Read the model definition and answer for the solid it produces. Units are mm, in the model's axes. Coordinates: 2 decimals unless noted, no trailing zeros. Write each loop counter-clockwise with the first axis right and the second up, starting at its lowest first coordinate (ties: lowest second). Pieces come first, ordered by that corner, then holes.
(1) Straight lines are drawn through the part: line 1 along Z through (x, y) = (2, 1.65); line 2 along Z through (x, y) = (52, 2.2); line 3 along X through (y, z) = (1.9, -65) (3 decimals). For each, find the intervals that lie inside material, in ascending order.
(2) The part is cut by section A-A, the plane x = 30. Determine the outline of the cut face in (y, z), and give its area (3 significant figures).
(3) The part is cut by section B-B, the plane y = 2.5. State how many separate pieces and enclosed holes the cut face has, and give its area (3 significant figures).
(4) The part is cut by section D-D, the plane x = 51. Determine the outline of the cut face in (y, z).
(5) The part is cut by section C-C, the plane z = 1. Determine the outline of the cut face in (x, y), and give its area (3 significant figures).
(6) Given pin 1 (9.5 mm diameter, centred on x = 60, z = -60, fed in from -Y); pin 2 (1.5 mm diameter, centred on y = 1, z = -28.5, fed in from -X), each flat-ended and moving along its own axis, determine where each tip first touches the part or whether it passes through.
```python
from build123d import *

# Parameters (mm, degrees)
SKETCH_1_R          = 8
SKETCH_1_W          = 60
SKETCH_1_H          = 60
SKETCH_1_R_2        = 20
SKETCH_1_R_3        = 1.75
EXTRUDE_1_DEPTH     = 3
FILLET_1_R          = 10
CUT_EXTRUDE_START   = -3
SKETCH_2_R          = 6
CUT_EXTRUDE_1_DEPTH = 2
SKETCH_2_3_R        = 3.5
CUT_EXTRUDE_3_DEPTH = 97.213304693
CUT_EXTRUDE_6_DEPTH = 1.5


with BuildPart() as part:
    # Эскиз1 → Бобышка-Вытянуть1 (new body)
    # profile 1 of 5: a face of its own
    with BuildSketch(Plane(origin=(0, 0, 0), x_dir=(1, 0, 0), z_dir=(0, 1, 0))):
        with Locations((60, 60)):
            Circle(SKETCH_1_R)
    # profile 2 of 5: a face of its own
    with BuildSketch(Plane(origin=(0, 0, 0), x_dir=(1, 0, 0), z_dir=(0, 1, 0))):
        with Locations((0, 60)):
            Circle(SKETCH_1_R)
    # profile 3 of 5: a face of its own
    with BuildSketch(Plane(origin=(0, 0, 0), x_dir=(1, 0, 0), z_dir=(0, 1, 0))):
        with Locations((60, 0)):
            Circle(SKETCH_1_R)
    # profile 4 of 5: a face of its own
    with BuildSketch(Plane(origin=(0, 0, 0), x_dir=(1, 0, 0), z_dir=(0, 1, 0))):
        Circle(SKETCH_1_R)
    # profile 5 of 5: a face of its own
    with BuildSketch(Plane(origin=(0, 0, 0), x_dir=(1, 0, 0), z_dir=(0, 1, 0))):
        with Locations((30, 30)):
            Rectangle(SKETCH_1_W, SKETCH_1_H)
        with Locations(Location((30, 30, 0), (0, 0, 270))):
            Circle(SKETCH_1_R_2, mode=Mode.SUBTRACT)
        with Locations(Location((9, 51, 0), (0, 0, 270))):
            Circle(SKETCH_1_R_3, mode=Mode.SUBTRACT)
        with Locations(Location((51, 51, 0), (0, 0, 270))):
            Circle(SKETCH_1_R_3, mode=Mode.SUBTRACT)
        with Locations(Location((51, 9, 0), (0, 0, 270))):
            Circle(SKETCH_1_R_3, mode=Mode.SUBTRACT)
        with Locations(Location((9, 9, 0), (0, 0, 270))):
            Circle(SKETCH_1_R_3, mode=Mode.SUBTRACT)
    extrude(amount=EXTRUDE_1_DEPTH)

    # Скругление1
    fillet_1_edges = [part.edges().sort_by_distance(p)[0] for p in [
        (0, 1.5, -8),
        (0, 1.5, -52),
        (8, 1.5, -60),
        (52, 1.5, -60),
        (60, 1.5, -52),
        (60, 1.5, -8),
        (52, 1.5, 0),
        (8, 1.5, 0),
    ]]
    fillet(fillet_1_edges, radius=FILLET_1_R)

    # Эскиз2 → Вырез-Вытянуть1 (cut)
    with BuildSketch(Plane(origin=(0, 3, 0), x_dir=(1, 0, 0), z_dir=(0, 1, 0)).offset(CUT_EXTRUDE_START)):
        with Locations(Location((0, 60, 0), (0, 0, 270))):
            Circle(SKETCH_2_R)
        with Locations(Location((60, 60, 0), (0, 0, 270))):
            Circle(SKETCH_2_R)
        with Locations(Location((60, 0, 0), (0, 0, 270))):
            Circle(SKETCH_2_R)
        with Locations(Location((0, 0, 0), (0, 0, 270))):
            Circle(SKETCH_2_R)
    extrude(amount=CUT_EXTRUDE_1_DEPTH, mode=Mode.SUBTRACT)

    # Эскиз2<3> → Вырез-Вытянуть3 (cut, through all)
    with BuildSketch(Plane(origin=(0, 3, 0), x_dir=(1, 0, 0), z_dir=(0, 1, 0))):
        with Locations(Location((0, 0, 0), (0, 0, 270))):
            Circle(SKETCH_2_3_R)
        with Locations(Location((0, 60, 0), (0, 0, 270))):
            Circle(SKETCH_2_3_R)
        with Locations(Location((60, 60, 0), (0, 0, 270))):
            Circle(SKETCH_2_3_R)
        with Locations(Location((60, 0, 0), (0, 0, 270))):
            Circle(SKETCH_2_3_R)
    extrude(amount=-CUT_EXTRUDE_3_DEPTH, mode=Mode.SUBTRACT)

    # Эскиз5 → Вырез-Вытянуть6 (cut)
    with BuildSketch(Plane(origin=(0, 3, 0), x_dir=(1, 0, 0), z_dir=(0, 1, 0)).offset(CUT_EXTRUDE_START)):
        with BuildLine():
            Line((24.5, 57.5), (35.5, 57.5))
            ThreePointArc((35.5, 57.5), (36.914213562, 56.914213562), (37.5, 55.5))
            Line((37.5, 55.5), (37.5, 54.5))
            ThreePointArc((37.5, 54.5), (36.914213562, 53.085786438), (35.5, 52.5))
            Line((35.5, 52.5), (24.5, 52.5))
            ThreePointArc((24.5, 52.5), (23.085786438, 53.085786438), (22.5, 54.5))
            Line((22.5, 54.5), (22.5, 55.5))
            ThreePointArc((22.5, 55.5), (23.085786438, 56.914213562), (24.5, 57.5))
        make_face()
        with BuildLine():
            Line((37.5, 4.5), (37.5, 5.5))
            ThreePointArc((37.5, 5.5), (36.914213562, 6.914213562), (35.5, 7.5))
            Line((35.5, 7.5), (24.5, 7.5))
            ThreePointArc((24.5, 7.5), (23.085786438, 6.914213562), (22.5, 5.5))
            Line((22.5, 5.5), (22.5, 4.5))
            ThreePointArc((22.5, 4.5), (23.085786438, 3.085786438), (24.5, 2.5))
            Line((24.5, 2.5), (35.5, 2.5))
            ThreePointArc((35.5, 2.5), (36.914213562, 3.085786438), (37.5, 4.5))
        make_face()
    extrude(amount=CUT_EXTRUDE_6_DEPTH, mode=Mode.SUBTRACT)


solid = part.part
```
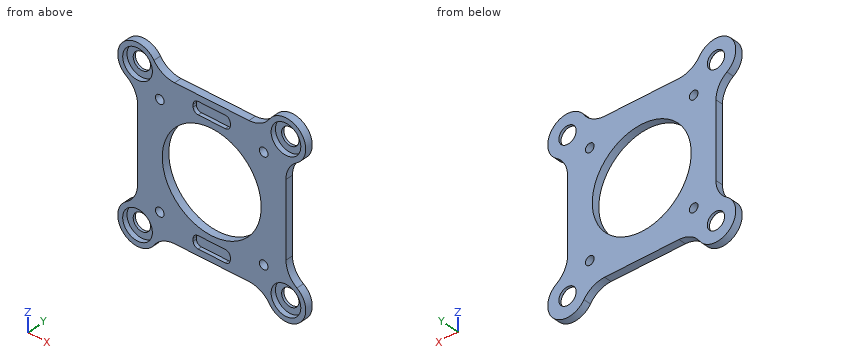
Computed:
1. line 1: z = -67.75 to -65.66, -54.34 to -5.66, 5.66 to 7.75
1. line 2: z = -62.83 to -52.44, -49.56 to -10.44, -7.56 to 2.83
1. line 3: x = -6.245 to -3.317, 3.317 to 6.245, 53.755 to 56.683, 63.317 to 66.245
2. outline: (0, -60) - (3, -60) - (3, -50) - (0, -50) - (0, -52.5) - (1.5, -52.5) - (1.5, -57.5) - (0, -57.5) - close; (0, -10) - (3, -10) - (3, 0) - (0, 0) - (0, -2.5) - (1.5, -2.5) - (1.5, -7.5) - (0, -7.5) - close
2. area: 45.0 mm2
3. separate pieces: 1
3. enclosed holes: 9
3. area: 2,810 mm2
4. outline: (0, -61.98) - (3, -61.98) - (3, -52.75) - (0, -52.75) - close; (0, -49.25) - (3, -49.25) - (3, -10.75) - (0, -10.75) - close; (0, -7.25) - (3, -7.25) - (3, 1.98) - (0, 1.98) - close
5. outline: (-7.94, 0) - (-5.92, 0) - (-5.92, 2) - (-3.35, 2) - (-3.35, 3) - (-7.94, 3) - close; (3.35, 2) - (5.92, 2) - (5.92, 0) - (10.61, 0) - (10.61, 3) - (3.35, 3) - close; (49.39, 0) - (54.08, 0) - (54.08, 2) - (56.65, 2) - (56.65, 3) - (49.39, 3) - close; (63.35, 2) - (65.92, 2) - (65.92, 0) - (67.94, 0) - (67.94, 3) - (63.35, 3) - close
5. area: 50.5 mm2
6. pin 1: stops at y = 2
6. pin 2: stops at x = 0
